Design review of the part built by this model. Coordinates are the model's own, in mm. Face numbers are marked on the shaded views. A direction names the side the tool comes from. Give positions to 0.01 mm unless a question says otherwise; leave off trailing zeros. Write each loop counter-clockwise with the first axis right and the second up, starting at its lowest first coordinate (ties: lowest second). Pieces come first, ordered by that corner, then holes. Notation, with made-up numbers: (34, -16.75) -> (45, -16.75) arc R20 cw to (45, -5.75) -> close; hole circle Ø6 at (11, 48). An arc over 180 degrees is marked (long way). Answer as a JSON object with one key per item and string values.
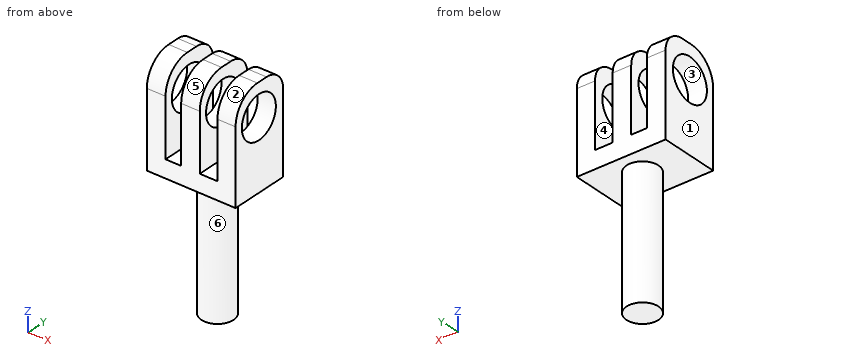
```python
from build123d import *

# Parameters (mm, degrees)
F0_W     = 4.6103289351
F0_H     = 4.3393736705
F0_W_2   = 3.8445899263
F0_H_2   = 20.9079552442
F0_W_3   = 4.5673176646
F0_H_3   = 20.7905257121
F0_W_4   = 4.3573188595
F0_W_5   = 4.4623203576
F0_H_4   = 20.6730971113
F1_DEPTH = 14.58655
F2_R     = 5.2152852963
F3_DEPTH = 26.42732
F4_R     = 6.6748900837
F5_R     = 5.08
F6_R     = 3.9375516614
F7_DEPTH = 31.84089


with BuildPart() as f1:
    # F0 (on Front) → F1 (new body)
    with BuildSketch(Plane.XZ):
        with Locations((-5.2306521684, -7.9293963499)):
            Rectangle(F0_W, F0_H)
        with Locations((-1.0031927377, -7.9293963499)):
            Rectangle(F0_W_2, F0_H)
        with Locations((-5.2306521684, 4.6942681074)):
            Rectangle(F0_W, F0_H_2)
        with Locations((3.2027610578, -7.9293963499)):
            Rectangle(F0_W_3, F0_H)
        with Locations((3.2027610578, 4.6355533414)):
            Rectangle(F0_W_3, F0_H_3)
        with Locations((7.6650793198, -7.9293963499)):
            Rectangle(F0_W_4, F0_H)
        with Locations((12.0748989284, -7.9293963499)):
            Rectangle(F0_W_5, F0_H)
        with Locations((12.0748989284, 4.576839041)):
            Rectangle(F0_W_5, F0_H_4)
    extrude(amount=F1_DEPTH)

    # F2 (on face) → F3 (cut)
    with BuildSketch(Plane.YZ.offset(14.3060591072)):
        with Locations((-7.4513442814, 6.9766114466)):
            Circle(F2_R)
    extrude(amount=-F3_DEPTH, mode=Mode.SUBTRACT)

    # F4
    f4_edges = [f1.edges().sort_by_distance(p)[0] for p in [
        (-5.230652, -14.58655, 15.148246),
        (3.202761, -14.58655, 15.030816),
        (12.074899, -14.58655, 14.913388),
    ]]
    fillet(f4_edges, radius=F4_R)

    # F5
    f5_edges = [f1.edges().sort_by_distance(p)[0] for p in [
        (12.074899, 0, 14.913388),
        (3.202761, 0, 15.030816),
        (-5.230652, 0, 15.148246),
    ]]
    fillet(f5_edges, radius=F5_R)

    # F6 (on face) → F7 (join)
    with BuildSketch(Plane(origin=(0, 0, -10.0990831852), x_dir=(1, 0, 0), z_dir=(0, 0, -1))):
        with Locations((3.3851212356, 6.5314560197)):
            Circle(F6_R)
    extrude(amount=F7_DEPTH)


solid = f1.part
```
(1) For line 1 along X through (y, z) = (-11.5, -4); line 2 along Z through (x, y) = (5.75, -9.5); line 3 along Z through (x, y) = (-2, -13.25), list the stretches that pass through material, from the lowest coordinate up.
Here are the results:
{"line 1": "x = -7.54 to -2.93, 0.92 to 5.49, 9.84 to 14.31", "line 2": "z = -41.94 to -5.76", "line 3": "z = -10.1 to -5.76"}
(2) We need section A-A, the plane z = -1.5. State the section outline as (x, y) points, then the cut area to 3 significant figures.
Here are the results:
{"outline": "(-7.54, -14.59) -> (-2.93, -14.59) -> (-2.93, 0) -> (-7.54, 0) -> close; (0.92, -14.59) -> (5.49, -14.59) -> (5.49, 0) -> (0.92, 0) -> close; (9.84, -14.59) -> (14.31, -14.59) -> (14.31, 0) -> (9.84, 0) -> close", "area": "199 mm²"}
(3) Clearance check with flat-ended pins moving along their axes: pin 1 (1.4 mm diameter, centred on x = 12.5, y = -7, fed in from +Z); pin 2 (2 mm diameter, centred on x = 4.5, y = -11.5, fed in from -Z); pin 3 (2 mm diameter, centred on x = 8, y = -4, fed in from +Z). State where each tip first meets the part, or that it passes through.
Here are the results:
{"pin 1": "stops at z = 14.91", "pin 2": "stops at z = -10.1", "pin 3": "stops at z = -5.76"}
(4) We need section B-B, the plane y = -6. State the section outline as (x, z) points.
Here are the results:
{"outline": "(-7.54, -10.1) -> (-0.52, -10.1) -> (-0.52, -41.94) -> (7.29, -41.94) -> (7.29, -10.1) -> (14.31, -10.1) -> (14.31, 1.97) -> (9.84, 1.97) -> (9.84, -5.76) -> (5.49, -5.76) -> (5.49, 1.97) -> (0.92, 1.97) -> (0.92, -5.76) -> (-2.93, -5.76) -> (-2.93, 1.97) -> (-7.54, 1.97) -> close; (-7.54, 11.99) -> (-2.93, 11.99) -> (-2.93, 15.15) -> (-7.54, 15.15) -> close; (0.92, 11.99) -> (5.49, 11.99) -> (5.49, 15.03) -> (0.92, 15.03) -> close; (9.84, 11.99) -> (14.31, 11.99) -> (14.31, 14.91) -> (9.84, 14.91) -> close"}
(5) For the marked faces 4, 5 and 6, list the 3-axis set-ups (+Z, -Z, +X, -X, +Y, -Y) from which the entire face can be reached by the end or side of a thin tool; tool diameter is ignored.
Here are the results:
{"face 4": "+Z, +Y, -Y", "face 5": "+Z, +X, -Y", "face 6": "-Z"}
(6) We need section C-C, the plane x = 12. State the section outline as (y, z) points.
Here are the results:
{"outline": "(-14.59, -10.1) -> (0, -10.1) -> (0, 9.83) arc R5.08 ccw to (-5.08, 14.91) -> (-7.91, 14.91) arc R6.67 ccw to (-14.59, 8.24) -> close; hole circle Ø10.43 at (-7.45, 6.98)"}
(7) The part is to be moulded in two halves that separate along Y. For the marked faces 1, 2 and 3, say which applies: +Y half, -Y half, draft (parallel to the pull), parting line (faces both ways), or undercut.
Here are the results:
{"face 1": "draft", "face 2": "-Y half", "face 3": "undercut"}
(8) We need section D-D, the plane z = 7.5. State the section outline as (x, y) points, then the cut area to 3 significant figures.
Here are the results:
{"outline": "(-7.54, -14.59) -> (-2.93, -14.59) -> (-2.93, -12.64) -> (-7.54, -12.64) -> close; (-7.54, -2.26) -> (-2.93, -2.26) -> (-2.93, 0) -> (-7.54, 0) -> close; (0.92, -14.59) -> (5.49, -14.59) -> (5.49, -12.64) -> (0.92, -12.64) -> close; (0.92, -2.26) -> (5.49, -2.26) -> (5.49, 0) -> (0.92, 0) -> close; (9.84, -14.59) -> (14.31, -14.59) -> (14.31, -12.64) -> (9.84, -12.64) -> close; (9.84, -2.26) -> (14.31, -2.26) -> (14.31, 0) -> (9.84, 0) -> close", "area": "57.4 mm²"}
